from build123d import *

# Parameters (mm, degrees)
SKETCH1_W           = 4.826
SKETCH1_H           = 25.4
BOSS_EXTRUDE1_DEPTH = 4.826
SKETCH2_W           = 25.4
SKETCH2_H           = 4.826
CUT_EXTRUDE1_DEPTH  = 5.826


with BuildPart() as part:
    # Sketch1 → Boss-Extrude1 (new body)
    with BuildSketch(Plane(origin=(0, 0, 0), x_dir=(1, 0, 0), z_dir=(0, 1, 0))):
        Polygon((0, 25.4), (0, 0), (622.3, 0), (622.3, 25.4), (617.474, 25.4), (617.474, 50.8), (622.3, 50.8), (622.3, 76.2), (617.474, 76.2), (617.474, 101.6), (622.3, 101.6), (622.3, 127), (0, 127), (0, 101.6), (4.826, 101.6), (4.826, 76.2), (0, 76.2), (0, 50.8), (4.826, 50.8), (4.826, 25.4), align=None)
        with Locations((92.837, 38.1)):
            Rectangle(SKETCH1_W, SKETCH1_H, mode=Mode.SUBTRACT)
        with Locations((529.463, 38.1)):
            Rectangle(SKETCH1_W, SKETCH1_H, mode=Mode.SUBTRACT)
        with Locations((92.837, 88.9)):
            Rectangle(SKETCH1_W, SKETCH1_H, mode=Mode.SUBTRACT)
        with Locations((529.463, 88.9)):
            Rectangle(SKETCH1_W, SKETCH1_H, mode=Mode.SUBTRACT)
    extrude(amount=BOSS_EXTRUDE1_DEPTH)

    # Sketch2 → Cut-Extrude1 (cut, through all)
    with BuildSketch(Plane(origin=(0, 4.826, 0), x_dir=(1, 0, 0), z_dir=(0, 1, 0))):
        with Locations((133.35, 124.587)):
            Rectangle(SKETCH2_W, SKETCH2_H)
        with Locations((184.15, 124.587)):
            Rectangle(SKETCH2_W, SKETCH2_H)
        with Locations((234.95, 124.587)):
            Rectangle(SKETCH2_W, SKETCH2_H)
        with Locations((285.75, 124.587)):
            Rectangle(SKETCH2_W, SKETCH2_H)
        with Locations((336.55, 124.587)):
            Rectangle(SKETCH2_W, SKETCH2_H)
        with Locations((387.35, 124.587)):
            Rectangle(SKETCH2_W, SKETCH2_H)
        with Locations((438.15, 124.587)):
            Rectangle(SKETCH2_W, SKETCH2_H)
        with Locations((488.95, 124.587)):
            Rectangle(SKETCH2_W, SKETCH2_H)
        with Locations((488.95, 2.413)):
            Rectangle(SKETCH2_W, SKETCH2_H)
        with Locations((438.15, 2.413)):
            Rectangle(SKETCH2_W, SKETCH2_H)
        with Locations((387.35, 2.413)):
            Rectangle(SKETCH2_W, SKETCH2_H)
        with Locations((336.55, 2.413)):
            Rectangle(SKETCH2_W, SKETCH2_H)
        with Locations((133.35, 2.413)):
            Rectangle(SKETCH2_W, SKETCH2_H)
        with Locations((184.15, 2.413)):
            Rectangle(SKETCH2_W, SKETCH2_H)
        with Locations((234.95, 2.413)):
            Rectangle(SKETCH2_W, SKETCH2_H)
        with Locations((285.75, 2.413)):
            Rectangle(SKETCH2_W, SKETCH2_H)
    extrude(amount=-CUT_EXTRUDE1_DEPTH, mode=Mode.SUBTRACT)


solid = part.part
The listing builds one solid part. Answer for the finished solid, in the listing's coordinates (mm). Coordinates: 2 decimals unless noted, no trailing zeros. Loops run counter-clockwise (first coordinate to the right, second up) from the corner with the lowest first, then second, coordinate; pieces in that order, holes last. Notation, with made-up numbers: (-32.75, 55.25) -> (-26.75, 55.25) arc R8 ccw to (-26.75, 64.25) -> close; hole circle Ø10 at (39.25, -2.75). An arc over 180 degrees is marked (long way). Write item = value, one per line. Start each with the question number.
1) Straight lines are drawn through the part: line 1 (X direction, y = 1.75, z = -88.5); line 2 (Z direction, x = 290.5, y = 1.85). For each, find the intervals that lie inside material, in ascending order. Write a range as from..to.
2) A cutting plane is placed at A-A (y = 4.1). Count the separate pieces of the cut face and the enclosed holes in it, then the cut area to 3 significant figures.
3) Given pin 1 Ø1 at (x, y) = (396, 0.5) entering from -Z; pin 2 Ø1.4 at (y, z) = (2, -85.5) entering from +X; pin 3 Ø1.5 at (x, y) = (233, 2) entering from +Z, each flat-ended and moving along its own axis, determine where each tip first touches the part or whether it passes through.
4) A cutting plane is placed at B-B (x = 190). Give the vertices of the cut face in (y, z).
Responses:
q1.line_1 = 4.83..90.42, 95.25..527.05, 531.88..617.47
q1.line_2 = -122.17..-4.83
q2.separate_pieces = 1
q2.enclosed_holes = 4
q2.area = 76,100 mm²
q3.pin_1 = -122.17
q3.pin_2 = 617.47
q3.pin_3 = -4.83
q4.outline = (0, -122.17) -> (4.83, -122.17) -> (4.83, -4.83) -> (0, -4.83) -> close
